Verification items for the finished model (mm, model axes). A direction names the side the tool comes from. Give positions to 0.01 mm unless a question says otherwise; leave off trailing zeros. Order: outer loops, then holes, each group sorted by start corner. A loop starts at its lowest first (then second) coordinate and runs counter-clockwise, first axis right, second up. Notation, with made-up numbers: M -14.5,17 L 36.5,17 A15 cw 36.5,22 Z; hole C 68,-1 d3. An arc over 180 degrees is marked long. Answer as a JSON object with one key per item and string values.
```python
from build123d import *

# Parameters (mm, degrees)
SKETCH007_R      = 1.5
EXTRUDE012_DEPTH = 75
SKETCH008_R      = 13
EXTRUDE014_DEPTH = 3.5
EXTRUDE002_DEPTH = 44
SKETCH002_W      = 3.5
SKETCH002_H      = 8
EXTRUDE003_DEPTH = 75
SKETCH003_W      = 40
SKETCH003_H      = 10
EXTRUDE005_DEPTH = 30
SKETCH004_W      = 68.5
SKETCH004_H      = 30
EXTRUDE006_DEPTH = 6
SKETCH005_W      = 5.5
SKETCH005_H      = 24
EXTRUDE008_DEPTH = 12
EXTRUDE009_DEPTH = 3
EXTRUDE010_DEPTH = 3
EXTRUDE_DEPTH    = 9


with BuildPart() as extrude012:
    # Sketch007 → Extrude012 (new body)
    with BuildSketch(Plane.XY):
        with Locations((-45, 23)):
            Circle(SKETCH007_R)
        with Locations((45, 23)):
            Circle(SKETCH007_R)
    extrude(amount=EXTRUDE012_DEPTH)


with BuildPart() as extrude014:
    # Sketch008 → Extrude014 (new body)
    with BuildSketch(Plane.XY):
        with Locations((-45, 23)):
            Circle(SKETCH008_R)
        with Locations((45, 23)):
            Circle(SKETCH008_R)
    extrude(amount=EXTRUDE014_DEPTH)


with BuildPart() as extrude002:
    # Sketch001 (on Face6 of Extrude) → Extrude002 (new body)
    with BuildSketch(Plane.XY.offset(9)):
        with BuildLine():
            Line((-14, 21), (-14, -1))
            ThreePointArc((-14, -1), (-10.485281, -9.485281), (-2, -13))
            Line((-2, -13), (2, -13))
            ThreePointArc((2, -13), (10.485281, -9.485281), (14, -1))
            Line((14, 21), (14, -1))
            Line((-14, 21), (14, 21))
        make_face()
    extrude(amount=EXTRUDE002_DEPTH)


with BuildPart() as extrude003:
    # Sketch002 (on Face6 of Extrude) → Extrude003 (new body)
    with BuildSketch(Plane.XY.offset(9)):
        with Locations((-17.75, 7)):
            Rectangle(SKETCH002_W, SKETCH002_H)
        with Locations((17.75, 7)):
            Rectangle(SKETCH002_W, SKETCH002_H)
    extrude(amount=EXTRUDE003_DEPTH)


with BuildPart() as extrude005:
    # Sketch003 (on Face6 of Extrude) → Extrude005 (new body)
    with BuildSketch(Plane.XY.offset(9)):
        with Locations((0, 7)):
            Rectangle(SKETCH003_W, SKETCH003_H)
    extrude(amount=EXTRUDE005_DEPTH)


with BuildPart() as extrude006:
    # Sketch004 → Extrude006 (new body)
    with BuildSketch(Plane.XY):
        with Locations((0, 24)):
            Rectangle(SKETCH004_W, SKETCH004_H)
    extrude(amount=EXTRUDE006_DEPTH)


with BuildPart() as extrude008:
    # Sketch005 (on Face6 of Extrude) → Extrude008 (new body)
    with BuildSketch(Plane.XY.offset(9)):
        with Locations((-2.75, 12)):
            Rectangle(SKETCH005_W, SKETCH005_H)
    extrude(amount=EXTRUDE008_DEPTH)


with BuildPart() as extrude009:
    # Sketch006 → Extrude009 (new body)
    with BuildSketch(Plane.XY):
        with BuildLine():
            ThreePointArc((-23.5, 92), (-27.742641, 90.242641), (-29.5, 86))
            Line((-29.5, 48), (-29.5, 86))
            ThreePointArc((-29.5, 48), (-27.742641, 43.757359), (-23.5, 42))
            Line((23.5, 42), (-23.5, 42))
            ThreePointArc((23.5, 42), (27.742641, 43.757359), (29.5, 48))
            Line((29.5, 86), (29.5, 48))
            ThreePointArc((29.5, 86), (27.742641, 90.242641), (23.5, 92))
            Line((-23.5, 92), (23.5, 92))
        make_face()
    extrude(amount=EXTRUDE009_DEPTH)


with BuildPart() as extrude010:
    # Sketch006 → Extrude010 (new body)
    with BuildSketch(Plane.XY):
        with BuildLine():
            ThreePointArc((-23.5, 92), (-27.742641, 90.242641), (-29.5, 86))
            Line((-29.5, 48), (-29.5, 86))
            ThreePointArc((-29.5, 48), (-27.742641, 43.757359), (-23.5, 42))
            Line((23.5, 42), (-23.5, 42))
            ThreePointArc((23.5, 42), (27.742641, 43.757359), (29.5, 48))
            Line((29.5, 86), (29.5, 48))
            ThreePointArc((29.5, 86), (27.742641, 90.242641), (23.5, 92))
            Line((-23.5, 92), (23.5, 92))
        make_face()
    extrude(amount=EXTRUDE010_DEPTH)


with BuildPart() as fusion001:
    # Sketch → Extrude (new body)
    with BuildSketch(Plane.XY):
        with BuildLine():
            ThreePointArc((-31.25, -1), (0, -13), (31.25, -1))
            Line((31.25, -1), (31.25, 47.5))
            Line((-31.25, 47.5), (31.25, 47.5))
            Line((-31.25, -1), (-31.25, 47.5))
        make_face()
    extrude(amount=EXTRUDE_DEPTH)

    # Fusion: union Extrude002, Extrude003, Extrude005, Extrude006, Extrude008, Extrude009, Extrude010
    add(extrude002.part)
    add(extrude003.part)
    add(extrude005.part)
    add(extrude006.part)
    add(extrude008.part)
    add(extrude009.part)
    add(extrude010.part)

    # Fusion001: union Extrude012, Extrude014
    add(extrude012.part)
    add(extrude014.part)


solid = fusion001.part
```
Q1. Gauge pin test, flat ends, axial feed: pin 1 Ø3 at (x, z) = (18, 20.5) entering from +Y; pin 2 Ø3 at (x, y) = (-17.5, 49.5) entering from +Z; pin 3 Ø1 at (y, z) = (11, 72.5) entering from -X. Record the tip position at first contact, or that the pin passes through.
Resolved:
{"pin 1": "stops at y = 12", "pin 2": "stops at z = 3", "pin 3": "stops at x = -19.5"}
Q2. Release check for a two-part mould opening along X. For faces 4 (the face through (-15.7, 7.1, 39)), 5 (the face through (-17, 12, 24)), 6 (the face through (29.5, 67, 1)) record: +X half, -X half, draft (parallel to the pull), parting line (faces both ways), or undercut.
Resolved:
{"face 4": "undercut", "face 5": "draft", "face 6": "+X half"}
Q3. Section check B-B on z = 17. Record the cut outline in (x, y), then the cut area to 3 significant figures.
Resolved:
{"outline": "C -45,23 d3; M -20,2 L -14,2 L -14,-1 A12 ccw -2,-13 L 2,-13 A12 ccw 14,-1 L 14,2 L 20,2 L 20,12 L 14,12 L 14,21 L 0,21 L 0,24 L -5.5,24 L -5.5,21 L -14,21 L -14,12 L -20,12 Z; C 45,23 d3", "area": "1,040 mm²"}
Q4. Section check D-D on z = 67.5. Record the cut outline in (x, y).
Resolved:
{"outline": "C -45,23 d3; M -19.5,3 L -16,3 L -16,11 L -19.5,11 Z; M 16,3 L 19.5,3 L 19.5,11 L 16,11 Z; C 45,23 d3"}
Q5. Section check C-C on x = 45. Record the cut outline in (y, z), then the cut area to 4 significant figures.
Resolved:
{"outline": "M 10,0 L 36,0 L 36,3.5 L 24.5,3.5 L 24.5,75 L 21.5,75 L 21.5,3.5 L 10,3.5 Z", "area": "305.5 mm²"}
Q6. Tool access check on faces 1 (the face through (-18, 7, 84)), 2 (the face through (-33, 9, 3)), 3 (the face through (20, 7, 24)). Record the directions out of +Z, -Z, +X, -X, +Y, -Y that give a thin tool (end or side, any length) a straight path to the whole face; none if there is none.
Resolved:
{"face 1": "+Z, +X, -X, +Y, -Y", "face 2": "+Z, -Z, -X, -Y", "face 3": "+Z, +X, +Y, -Y"}
Q7. Section check A-A on z = 47.5. Record the cut outline in (x, y), then the cut area to 3 significant figures.
Resolved:
{"outline": "C -45,23 d3; M -19.5,3 L -16,3 L -16,11 L -19.5,11 Z; M -14,-1 A12 ccw -2,-13 L 2,-13 A12 ccw 14,-1 L 14,21 L -14,21 Z; M 16,3 L 19.5,3 L 19.5,11 L 16,11 Z; C 45,23 d3", "area": "960 mm²"}
Q8. Material ranges on L1, parallel to Y at x = -0.5, z = 43; L2, parallel to X at y = 10.5, z = 32; L3, parallel to Z at x = -22.5, y = 65.5, recorded low to high.
Resolved:
{"L1": "y = -13 to 21", "L2": "x = -20 to 20", "L3": "z = 0 to 3"}
